```python
from build123d import *

# Parameters (mm, degrees)
F1_DEPTH = 10
F2_T     = 1


with BuildPart() as f1:
    # F0 (on Front) → F1 (new body)
    with BuildSketch(Plane.XZ):
        Polygon((-33.2895902376, 22.4671012992), (-36.3039637367, 17.568745036), (-33.0530058498, 12.8241044288), (-27.3014546092, 12.8241044288), (-24.2870811101, 17.7224606921), (-27.538038997, 22.4671012992), align=None)
    extrude(amount=F1_DEPTH)

    # F2
    f2_openings = [f1.faces().sort_by_distance(p)[0] for p in [
        (-30.295522, -10, 17.645603),
    ]]
    offset(amount=F2_T, openings=f2_openings, kind=Kind.INTERSECTION)


solid = f1.part
```
Design review of the part built by this model. Coordinates are the model's own, in mm. A direction names the side the tool comes from. Coordinates: 2 decimals unless noted, no trailing zeros. Write each loop counter-clockwise with the first axis right and the second up, starting at its lowest first coordinate (ties: lowest second). Pieces come first, ordered by that corner, then holes. Notation, with made-up numbers: M -28,8.5 L 26,8.5 A21 ccw 26,18.5 Z; hole C 23,17.25 d5. An arc over 180 degrees is marked long. Answer as a JSON object with one key per item and string values.
Item 1: Add section A-A, the plane y = -7.75. Give the boundary of the cut face in (x, z).
Outcome:
{"outline": "M -37.5,17.54 L -33.58,11.82 L -26.74,11.82 L -23.09,17.75 L -27.01,23.47 L -33.85,23.47 Z; hole M -36.3,17.57 L -33.05,12.82 L -27.3,12.82 L -24.29,17.72 L -27.54,22.47 L -33.29,22.47 Z"}
Item 2: Machinability: for faces 4 (the flat face through (-35.566, -4.423, 14.722)), 5 (the flat face through (-34.776, -4.93, 20.052)), which of the approach directions +Z, -Z, +X, -X, +Y, -Y give a long, thin tool a straight path to every point of the face, cutting with its end or side? Answer none if there is none.
Outcome:
{"face 4": "-Z, -X, +Y, -Y", "face 5": "-Y"}
Item 3: Insertion check: pin 1 Ø1.5 at (x, z) = (-31, 20) entering from -Y; pin 2 Ø1 at (y, z) = (-0.5, 15) entering from -X. Each pin has a flat end and moves straight along its axis. Give the tip position at first contact, or say it passes through.
Outcome:
{"pin 1": "y = 0", "pin 2": "x = -36.1"}
Item 4: Add section B-B, the plane x = -25. Give the boundary of the cut face in (y, z).
Outcome:
{"outline": "M -10,14.66 L 1,14.66 L 1,20.53 L -10,20.53 L -10,18.76 L 0,18.76 L 0,16.56 L -10,16.56 Z"}
Item 5: Add section C-C, the plane z = 17. Give the boundary of the cut face in (x, y), and give its area (3 significant figures).
Outcome:
{"outline": "M -37.13,-10 L -35.91,-10 L -35.91,0 L -24.73,0 L -24.73,-10 L -23.56,-10 L -23.56,1 L -37.13,1 Z", "area": "37.4 mm²"}
Item 6: Wall thickness on probe 1 along Z at (x, y) = (-28.5, -7.75); probe 2 along Y at (x, z) = (-35.5, 17.25); probe 3 along Z at (x, y) = (-34.75, -1.75): over which ranges is each line inside the solid? List them lowest first.
Outcome:
{"probe 1": "11.82 to 12.82, 22.47 to 23.47", "probe 2": "0 to 1", "probe 3": "13.53 to 15.3, 20.09 to 22"}
Item 7: Draft analysis for pull direction Z (two halves, no side actions). For faces 1 (the flat face through (-30, 1, 18)), 2 (the flat face through (-30, -4, 23.467)), 3 (the flat face through (-34.7, -4.93, 15.23)), state which applies: pulls with the +Z half, pulls with the -Z half, needs draft (parallel to the pull), parting line crosses it, or undercut.
Outcome:
{"face 1": "needs draft", "face 2": "pulls with the +Z half", "face 3": "undercut"}
